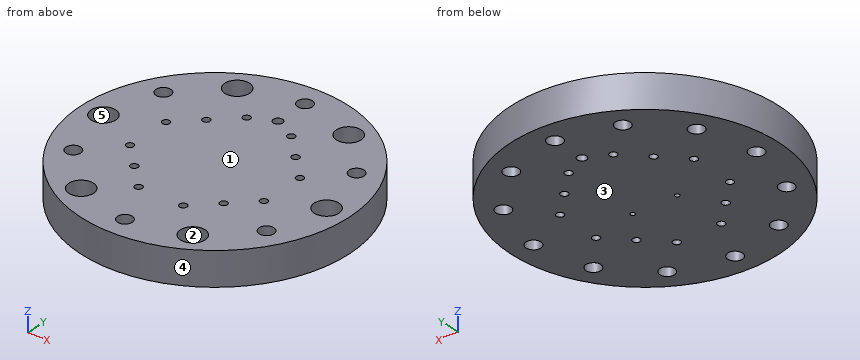
Autodesk Inventor part; units mm, degrees
ref_plane "YZ Plane" through (0, 0, 0) normal (1, 0, 0) x (0, 1, 0)
ref_plane "XZ Plane" through (0, 0, 0) normal (0, 1, 0) x (-1, 0, 0)
ref_plane "XY Plane" through (0, 0, 0) normal (0, 0, 1) x (1, 0, 0)
sketch "Sketch1" plane through (0, 0, 0) normal (0, 0, 1) x (1, 0, 0)
  circle A0 centre (0, 0) radius 60
  point P0 (0, 0)
  point P1 (-51.3571, -31.5041)
  point P2 (-31.5041, -51.3571)
extrude "Extrusion1" add sketch "Sketch1" along normal blind 15
sketch "Sketch13" plane through (0, 0, 0) normal (0, 0, -1) x (-1, 0, 0)
  point P0 (0, 0)
  point P1 (0, 0)
sketch "Sketch14" plane through (0, 0, 15) normal (0, 0, 1) x (1, 0, 0)
  circle A0 centre (0, 50) radius 2.4585
  point P0 (0, 0)
hole "Hole10" at (0, 50, 15) direction (0, 0, -1) diameter 6.6 depth 17.1
pattern_circular "Circular Pattern6" count 6 over 360 about axis through (0, 0, 0) along (0, 0, 1) of "Hole10"
sketch "Sketch15" plane through (0, 0, 15) normal (0, 0, 1) x (1, 0, 0)
  circle A0 centre (25, 43.3013) radius 2.4585
  point P0 (0, 0)
hole "Hole11" at (25, 43.3013, 15) direction (0, 0, -1) diameter 6.6 end through all counterbore diameter 11 counterbore depth 6.8
pattern_circular "Circular Pattern7" count 6 over 360 about axis through (0, 0, 0) along (0, 0, 1) of "Hole11"
sketch "Sketch16" plane through (0, 0, 0) normal (0, 0, -1) x (-1, 0, 0)
  line L0 (12.05, -6.95) -> (12.05, -3.5)
  line L1 (12.05, -3.5) -> (13, -3.5)
  line L2 (13, -3.5) -> (13, 6)
  line L3 (7, 12) -> (13, 6)
  line L4 (7, 12) -> (-7, 12)
  line L5 (-13, 6) -> (-7, 12)
  line L6 (-13, 6) -> (-13, -3.5)
  line L7 (-13, -3.5) -> (-12.05, -3.5)
  line L8 (-12.05, -3.5) -> (-12.05, -6.95)
  line L9 (-7, -12) -> (-12.05, -6.95)
  line L10 (-7, -12) -> (7, -12)
  line L11 (12.05, -6.95) -> (7, -12)
  circle A0 centre (-10, -5.5) radius 1.35
  circle A1 centre (10, -5.5) radius 1.35
  circle A2 centre (-10, 5.5) radius 0.8
  circle A3 centre (10, 5.5) radius 0.8
  point P0 (0, 0)
hole "Hole12" at (10, -5.5, 0) at (-10, -5.5, 0) direction (0, 0, 1) diameter 2.013 depth 7.6 tip angle 118
sketch "Sketch17" plane through (0, 0, 0) normal (0, 0, -1) x (-1, 0, 0)
  circle A0 centre (-10, 5.5) radius 0.8
  circle A1 centre (10, 5.5) radius 0.8
  point P0 (0, 0)
hole "Hole13" [suppressed]
sketch "Sketch18" plane through (0, 0, 0) normal (0, 0, -1) x (-1, 0, 0)
  circle A0 centre (0, 0) radius 40
  circle A1 centre (0, 0) radius 30
  line L0 (0, 30) -> (0, 40) construction
  circle A2 centre (0, 35) radius 2.5
  point P0 (0, 0)
  dimension "d114" = 5
hole "Hole14" at (0, 35, 0) direction (0, 0, 1) diameter 4.134 end through all
sketch "Sketch20" plane through (0, 0, 0) normal (0, 0, -1) x (-1, 0, 0)
  line L0 (-20, 20) -> (20, 20)
  line L1 (20, 20) -> (20, -20)
  line L2 (20, -20) -> (-20, -20)
  line L3 (-20, -20) -> (-20, 20)
  line L4 (-10, 30) -> (10, 30)
  line L5 (10, 30) -> (10, -30)
  line L6 (10, -30) -> (-10, -30)
  line L7 (-10, -30) -> (-10, 30)
  line L8 (-30, 10) -> (30, 10)
  line L9 (30, 10) -> (30, -10)
  line L10 (30, -10) -> (-30, -10)
  line L11 (-30, -10) -> (-30, 10)
  point P0 (0, 0)
  point P1 (0, 20)
  point P2 (-20, 0)
  point P3 (-20, 0)
  point P4 (0, 20)
  point P5 (20, 0)
  point P6 (0, -20)
  point P7 (-10, 0)
  point P8 (0, 30)
  point P9 (-30, 0)
  point P10 (0, 10)
  dimension "d124" = 40
  dimension "d125" = 40
  dimension "d141" = 60
  dimension "d142" = 20
  dimension "d143" = 20
  dimension "d144" = 60
hole "Hole15" at (20, 20, 0) at (-20, 20, 0) at (-20, -20, 0) at (20, -20, 0) at (30, -10, 0) at (30, 10, 0) at (10, 30, 0) at (-10, 30, 0) at (-30, 10, 0) at (-30, -10, 0) at (-10, -30, 0) at (10, -30, 0) direction (0, 0, 1) diameter 3.3 depth 20 tip angle 118
thread "Thread1"
thread "Thread2"
thread "Thread3"
thread "Thread4"
thread "Thread5"
thread "Thread6"
thread "Thread7"
thread "Thread8"
thread "Thread9"
thread "Thread10"
thread "Thread11"
thread "Thread12"
properties part number "base_becherboden" material "ABS Plastic"
The model under review builds one solid part; all positions refer to its coordinate system, in mm. Face numbers are marked on the shaded views. A direction names the side the tool comes from. Round coordinates to 2 decimals unless told otherwise and drop trailing zeros. Loops run counter-clockwise (first coordinate to the right, second up) from the corner with the lowest first, then second, coordinate; pieces in that order, holes last. Notation, with made-up numbers: M 52.5,72 L 100.5,72 A27 cw 100.5,99 Z; hole C -5,0.25 d9. An arc over 180 degrees is marked long. Answer as CSV lines item,"result". Start each with the question number.
Item 1: Mouldability with a two-part tool opening along X and no side actions: class the marked faces 3, 4 and 5 as released by +X, released by -X, zero draft, split by the parting line, or undercut.
Item 2: Consider section C-C (x = -50). Write out the cut boundary in (y, z).
Item 3: Wall thickness on line 1 (Y direction, x = -22.5, z = 6.25); line 2 (Y direction, x = -10, z = 10); line 3 (X direction, y = -5.5, z = 5.75): over which ranges is each line inside the solid? List them lowest first. Write a range as [from, to].
Item 4: Insertion check: P1, Ø5.5, axis at x = -10, y = 30, coming from the -Z side; P2, Ø1.5, axis at x = 26, z = 13, coming from the -Y side; P3, Ø1, axis at x = -8, z = 13, coming from the -Y side; P4, Ø2, axis at x = 9.5, z = 12.5, coming from the +Y side. Each pin has a flat end and moves straight along its axis. Give the tip position at first contact, or say it passes through.
Item 5: Consider section B-B (y = -20). Write out the cut boundary in (x, z).
Item 6: Consider section A-A (x = 0). Write out the cut boundary in (y, z), then the cut area to 3 significant figures.
Item 7: For the marked faces 1 and 2, list the 3-axis set-ups (+Z, -Z, +X, -X, +Y, -Y) from which the entire face can be reached by the end or side of a thin tool; tool diameter is ignored.
Item 8: Consider section D-D (y = 35). Write out the cut boundary in (x, z), then the cut area to 3 significant figures.
Answer:
1,face 3,"zero draft"
1,face 4,"split by the parting line"
1,face 5,"undercut"
2,outline,"M -33.17,0 L -3.3,0 L -3.3,8.2 L -5.5,8.2 L -5.5,15 L -33.17,15 Z; M 3.3,0 L 33.17,0 L 33.17,15 L 5.5,15 L 5.5,8.2 L 3.3,8.2 Z"
3,line 1,"y = [-55.62, -45.46], [-41.15, 41.15], [45.46, 55.62]"
3,line 2,"y = [-59.16, -31.65], [-28.35, 28.35], [31.65, 59.16]"
3,line 3,"x = [-59.75, -11.01], [-8.99, 8.99], [11.01, 59.75]"
4,P1,"stops at z = 0"
4,P2,"stops at y = -54.43"
4,P3,"stops at y = -59.53"
4,P4,"stops at y = 59.39"
5,outline,"M -56.57,0 L -21.65,0 L -21.65,15 L -56.57,15 Z; M -18.35,0 L 18.35,0 L 18.35,15 L -18.35,15 Z; M 21.65,0 L 56.57,0 L 56.57,15 L 21.65,15 Z"
6,outline,"M -60,0 L -53.3,0 L -53.3,15 L -60,15 Z; M -46.7,0 L 32.93,0 L 32.93,15 L -46.7,15 Z; M 37.07,0 L 46.7,0 L 46.7,15 L 37.07,15 Z; M 53.3,0 L 60,0 L 60,15 L 53.3,15 Z"
6,area,"1,540 mm^2"
7,face 1,"+Z, +X, -X, +Y, -Y"
7,face 2,"+Z"
8,outline,"M -48.73,0 L -2.07,0 L -2.07,15 L -48.73,15 Z; M 2.07,0 L 48.73,0 L 48.73,15 L 2.07,15 Z"
8,area,"1,400 mm^2"
